Can you work these out from the model? Positions are in its coordinate system, mm. A direction names the side the tool comes from. Give positions to 0.01 mm unless a question says otherwise; leave off trailing zeros. Loops run counter-clockwise (first coordinate to the right, second up) from the corner with the lowest first, then second, coordinate; pieces in that order, holes last. Notation, with made-up numbers: (-29, 50.25) - (24, 50.25) arc R37 ccw to (24, 86.25) - close; hole circle Ø6 at (-31.5, 61.5). An arc over 180 degrees is marked (long way). Answer in a Markdown table with one row per item.
from build123d import *

# Parameters (mm, degrees)
F0_R     = 1.575
F1_DEPTH = 30
F3_D     = 1.75
F3_DEPTH = 6
F3_TIP   = 0.5257530416
F5_D     = 1.75
F5_DEPTH = 6
F5_TIP   = 0.5257530416


with BuildPart() as f1:
    # F0 (on Top) → F1 (new body)
    with BuildSketch(Plane.XY):
        Circle(F0_R)
    extrude(amount=F1_DEPTH)

    # F3
    with Locations(Plane.XY.offset(30)):
        with Locations((0, 0)):
            Hole(F3_D / 2, depth=F3_DEPTH)
            with Locations((0, 0, -(F3_DEPTH + F3_TIP / 2))):  # 118° drill point
                Cone(0, F3_D / 2, F3_TIP, mode=Mode.SUBTRACT)

    # F5
    with Locations(Plane(origin=(0, 0, 0), x_dir=(1, 0, 0), z_dir=(0, 0, -1))):
        with Locations((0, 0)):
            Hole(F5_D / 2, depth=F5_DEPTH)
            with Locations((0, 0, -(F5_DEPTH + F5_TIP / 2))):  # 118° drill point
                Cone(0, F5_D / 2, F5_TIP, mode=Mode.SUBTRACT)


solid = f1.part
Q1. If we mould it in two halves opening along X, with no side actions, what happens to faces 3 (the face through (-1.25, -0.96, 14.79)), 4 (the face through (1, -1, 30)), 5 (the face through (-0.808, 0.335, 3.042))? For each: released by +X, released by -X, zero draft, split by the parting line, or undercut.
Checked values:
| item | result |
|---|---|
| face 3 | split by the parting line |
| face 4 | zero draft |
| face 5 | undercut |
Q2. If I drill on line 1 (Y direction, x = 0, z = 3.45) (3 decimals); line 2 (X direction, y = 0.1, z = 2.5); line 3 (Y direction, x = -0.55, z = 4.5), over which ranges is the centre line in solid material (lowest first)? Write a range as [from, to].
Checked values:
| item | result |
|---|---|
| line 1 | y = [-1.575, -0.875], [0.875, 1.575] |
| line 2 | x = [-1.57, -0.87], [0.87, 1.57] |
| line 3 | y = [-1.48, -0.68], [0.68, 1.48] |
Q3. For pin 1 (1.6 mm diameter, centred on x = 0, y = 0, fed in from -Z), with a flat end and sliding along its axis, tell me the tip position at first contact or that it passes through.
Checked values:
| item | result |
|---|---|
| pin 1 | stops at z = 6.05 |
Q4. Imagine slicing it at A-A, the plane z = 2.5. Write out the boundary of the cut face in (x, y) (3 decimals), and give its area (3 significant figures).
Checked values:
| item | result |
|---|---|
| outline | circle Ø3.15 at (0, 0); hole circle Ø1.75 at (0, 0) |
| area | 5.39 mm² |
Q5. Imagine slicing it at C-C, the plane y = 1.25. Write out the boundary of the cut face in (x, z).
Checked values:
| item | result |
|---|---|
| outline | (-0.96, 0) - (0.96, 0) - (0.96, 30) - (-0.96, 30) - close |
Q6. On a 3-axis mill with a long thin cutter (end or side, diameter ignored), from which of +Z, -Z, +X, -X, +Y, -Y can I reach the whole of each face in a straight line? I mean faces 1 (the face through (-0.033, 0.148, 6.434)), 2 (the face through (-0.808, -0.335, 26.958)). Say none if no direction works.
Checked values:
| item | result |
|---|---|
| face 1 | -Z |
| face 2 | +Z |
Q7. Imagine slicing it at B-B, the plane z = 10.5. Write out the boundary of the cut face in (x, y) (3 decimals), and give its area (3 significant figures).
Checked values:
| item | result |
|---|---|
| outline | circle Ø3.15 at (0, 0) |
| area | 7.79 mm² |
Q8. Imagine slicing it at D-D, the plane x = -1.15. Write out the boundary of the cut face in (y, z), and give its area (3 significant figures).
Checked values:
| item | result |
|---|---|
| outline | (-1.08, 0) - (1.08, 0) - (1.08, 30) - (-1.08, 30) - close |
| area | 64.6 mm² |
